Design review of the part built by this model. Coordinates are the model's own, in mm. Face numbers are marked on the shaded views. A direction names the side the tool comes from. Coordinates: 2 decimals unless noted, no trailing zeros. Loops run counter-clockwise (first coordinate to the right, second up) from the corner with the lowest first, then second, coordinate; pieces in that order, holes last. Notation, with made-up numbers: M 45,52 L 76,52 A11 cw 76,62 Z; hole C 69,87 d1. An arc over 180 degrees is marked long. Answer as a JSON object with one key per item and string values. Group by question number.
1. Insertion check: pin 1 (2.5 mm diameter, centred on x = 44.5, y = 8, fed in from -Z); pin 2 (4 mm diameter, centred on x = 61.5, y = 2.5, fed in from +Z); pin 3 (1.5 mm diameter, centred on x = 51, y = -5.5, fed in from -Z). Each pin has a flat end and moves straight along its axis. Give the tip position at first contact, or say it passes through.
2. Consider section C-C (x = 25). State the section outline as (y, z) points, then the cut area to 3 significant figures.
3. Consider section B-B (y = -4.5). State the section outline as (x, z) points.
4. Machinability: for the marked faces 1, 2, 3 and 4, which of the approach directions +Z, -Z, +X, -X, +Y, -Y give a long, thin tool a straight path to every point of the face, cutting with its end or side? Answer none if there is none.
5. Consider section A-A (x = 42). State the section outline as (y, z) points, then the cut area to 3 significant figures.
6. To check wall thickness, follow probe 1 along X at (y, z) = (4.75, 4.5); probe 2 along Z at (x, y) = (21.5, -2.25); probe 3 along Y at (x, z) = (57, -2.75). State the ranges of each line that lie inside material, in increasing order.
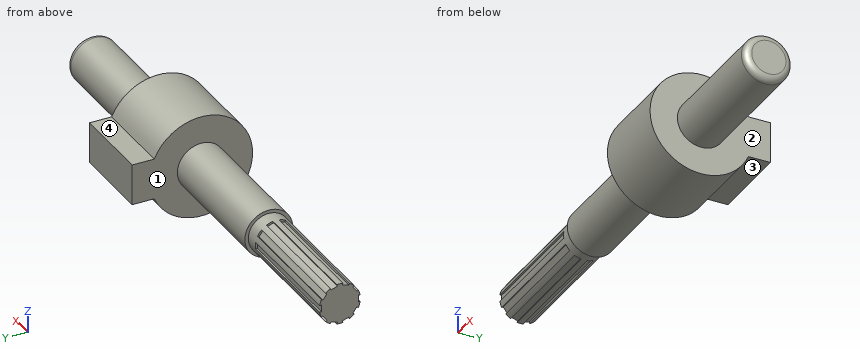
from build123d import *

# Parameters (mm, degrees)
Y_KSEKLIK_EKSTR_ZYON2_START = -12
Y_KSEKLIK_EKSTR_ZYON2_DEPTH = 12
KES_EKSTR_ZYON1_DEPTH       = 18
IZIM4_R                     = 3.5
IZIM4_R_2                   = 3
KES_EKSTR_ZYON2_DEPTH       = 20


with BuildPart() as part:
    # Çizim1 → Döndür1 (revolve)
    with BuildSketch(Plane.XY, mode=Mode.PRIVATE) as d_nd_r1_sk:
        with BuildLine():
            Line((0, 0), (70, 0))
            Line((70, 0), (70, 2.5))
            ThreePointArc((70, 2.5), (69.707106781, 3.207106781), (69, 3.5))
            Line((69, 3.5), (51, 3.5))
            Line((51, 3.5), (51, 7.5))
            Line((51, 7.5), (39, 7.5))
            Line((39, 7.5), (39, 3.5))
            Line((39, 3.5), (0, 3.5))
            Line((0, 3.5), (0, 0))
        make_face()
    revolve(d_nd_r1_sk.sketch.rotate(Axis((0, 0, 0), (1, 0, 0)), 90), axis=Axis((0, 0, 0), (1, 0, 0)))

    # Çizim2 → Yükseklik-Ekstrüzyon2 (add)
    with BuildSketch(Plane(origin=(51, 0, 0), x_dir=(0, 0, -1), z_dir=(1, 0, 0)).offset(Y_KSEKLIK_EKSTR_ZYON2_START)):
        with BuildLine():
            Line((-3, 10.1), (3, 10.1))
            Line((3, 10.1), (3, 6.873863542))
            ThreePointArc((3, 6.873863542), (0, 7.5), (-3, 6.873863542))
            Line((-3, 6.873863542), (-3, 10.1))
        make_face()
    extrude(amount=Y_KSEKLIK_EKSTR_ZYON2_DEPTH)

    # Çizim3 → Kes-Ekstrüzyon1 (cut)
    with BuildSketch(Plane.ZY):
        with BuildLine():
            Line((1.182511684, 2.478238511), (1.991528678, 1.890453259))
            Line((1.991528678, 1.890453259), (2.440656339, 2.508624451))
            ThreePointArc((2.440656339, 2.508624451), (2.057248383, 2.83155948), (1.631639345, 3.096409703))
            Line((1.631639345, 3.096409703), (1.182511684, 2.478238511))
        make_face()
        with BuildLine():
            Line((-0.5, 3.464101615), (-0.5, 2.7))
            Line((-0.5, 2.7), (0.5, 2.7))
            Line((0.5, 2.7), (0.5, 3.464101615))
            ThreePointArc((0.5, 3.464101615), (0, 3.5), (-0.5, 3.464101615))
        make_face()
        with BuildLine():
            Line((2.413344097, 1.309874143), (2.722361091, 0.358817627))
            Line((2.722361091, 0.358817627), (3.449064911, 0.594938011))
            ThreePointArc((3.449064911, 0.594938011), (3.328697807, 1.08155948), (3.140047917, 1.545994527))
            Line((3.140047917, 1.545994527), (2.413344097, 1.309874143))
        make_face()
        with BuildLine():
            Line((2.722361091, -0.358817627), (2.413344097, -1.309874143))
            Line((2.413344097, -1.309874143), (3.140047917, -1.545994527))
            ThreePointArc((3.140047917, -1.545994527), (3.328697807, -1.08155948), (3.449064911, -0.594938011))
            Line((3.449064911, -0.594938011), (2.722361091, -0.358817627))
        make_face()
        with BuildLine():
            Line((1.991528678, -1.890453259), (1.182511684, -2.478238511))
            Line((1.182511684, -2.478238511), (1.631639345, -3.096409703))
            ThreePointArc((1.631639345, -3.096409703), (2.057248383, -2.83155948), (2.440656339, -2.508624451))
            Line((2.440656339, -2.508624451), (1.991528678, -1.890453259))
        make_face()
        with BuildLine():
            Line((0.5, -2.7), (-0.5, -2.7))
            Line((-0.5, -2.7), (-0.5, -3.464101615))
            ThreePointArc((-0.5, -3.464101615), (0, -3.5), (0.5, -3.464101615))
            Line((0.5, -3.464101615), (0.5, -2.7))
        make_face()
        with BuildLine():
            Line((-1.182511684, -2.478238511), (-1.991528678, -1.890453259))
            Line((-1.991528678, -1.890453259), (-2.440656339, -2.508624451))
            ThreePointArc((-2.440656339, -2.508624451), (-2.057248383, -2.83155948), (-1.631639345, -3.096409703))
            Line((-1.631639345, -3.096409703), (-1.182511684, -2.478238511))
        make_face()
        with BuildLine():
            Line((-2.413344097, -1.309874143), (-2.722361091, -0.358817627))
            Line((-2.722361091, -0.358817627), (-3.449064911, -0.594938011))
            ThreePointArc((-3.449064911, -0.594938011), (-3.328697807, -1.08155948), (-3.140047917, -1.545994527))
            Line((-3.140047917, -1.545994527), (-2.413344097, -1.309874143))
        make_face()
        with BuildLine():
            Line((-2.722361091, 0.358817627), (-2.413344097, 1.309874143))
            Line((-2.413344097, 1.309874143), (-3.140047917, 1.545994527))
            ThreePointArc((-3.140047917, 1.545994527), (-3.328697807, 1.08155948), (-3.449064911, 0.594938011))
            Line((-3.449064911, 0.594938011), (-2.722361091, 0.358817627))
        make_face()
        with BuildLine():
            Line((-1.991528678, 1.890453259), (-1.182511684, 2.478238511))
            Line((-1.182511684, 2.478238511), (-1.631639345, 3.096409703))
            ThreePointArc((-1.631639345, 3.096409703), (-2.057248383, 2.83155948), (-2.440656339, 2.508624451))
            Line((-2.440656339, 2.508624451), (-1.991528678, 1.890453259))
        make_face()
    extrude(amount=-KES_EKSTR_ZYON1_DEPTH, mode=Mode.SUBTRACT)

    # Çizim4 → Kes-Ekstrüzyon2 (cut)
    with BuildSketch(Plane.ZY):
        Circle(IZIM4_R)
        Circle(IZIM4_R_2, mode=Mode.SUBTRACT)
    extrude(amount=-KES_EKSTR_ZYON2_DEPTH, mode=Mode.SUBTRACT)


solid = part.part
Findings below:
{
 "1": {"pin 1": "stops at z = -3.27", "pin 2": "stops at z = 3.46", "pin 3": "stops at z = -5.8"},
 "2": {"outline": "C 0,0 d7", "area": "38.5 mm^2"},
 "3": {"outline": "M 39,-6 L 51,-6 L 51,6 L 39,6 Z"},
 "4": {"face 1": "-X", "face 2": "+X", "face 3": "-Z, +X, -X, +Y", "face 4": "+Z, +X, -X, +Y"},
 "5": {"outline": "M 6.87,-3 L 10.1,-3 L 10.1,3 L 6.87,3 A7.5 ccw long Z", "area": "194 mm^2"},
 "6": {"probe 1": "x = 39 to 51", "probe 2": "z = -2.68 to 2.68", "probe 3": "y = -2.17 to 2.17"}
}
